Geometry check sheet. Reference: the model listing, model coordinates, mm. Face numbers are marked on the shaded views. A direction names the side the tool comes from. Round coordinates to 2 decimals unless told otherwise and drop trailing zeros. Loops run counter-clockwise (first coordinate to the right, second up) from the corner with the lowest first, then second, coordinate; pieces in that order, holes last. Notation, with made-up numbers: (-5.75, -14.5) - (5.25, -14.5) arc R16 cw to (5.25, 7.5) - close; hole circle Ø5 at (0.5, 21). An arc over 180 degrees is marked (long way). Answer as CSV lines item,"result". Start each with the question number.
1) Cross-section at A-A on x = 0. Record the boundary of the cut face in (y, z) (3 decimals), and give its area (3 significant figures).
2) Cross-section at C-C on y = -13. Record the boundary of the cut face in (x, z) (3 decimals).
3) Cross-section at B-B on z = 0. Record the boundary of the cut face in (x, y) (3 decimals), and give its area (3 significant figures).
4) Depth check by flat-ended pin: P1, Ø12, axis at x = -41.5, z = 12, coming from the +Y side; P2, Ø3, axis at y = -86, z = -41, coming from the -X side; P3, Ø4, axis at x = -43.5, z = 35.5, coming from the -Y side; P4, Ø3, axis at x = -5, y = -139, coming from the -Z side. Enter the tip coordinate at first touch or a pass-through.
5) Cross-section at D-D on x = 44. State how many separate pieces and enclosed holes the cut face has, and give its area (3 significant figures).
6) Draft check along Y on the marked faces 3, 4 and 5. Enter one of: released by +Y, released by -Y, zero draft, split by the parting line, or undercut.
7) Access from +Z, -Z, +X, -X, +Y, -Y to the whole of each face (thin tool, end or side, straight path). Record for the marked faces 1 and 2.
8) Thickness scan on line 1 along X through (y, z) = (-18, 0) (3 decimals); line 2 along X through (y, z) = (-116.2, 0) (3 decimals); line 3 along Y through (x, z) = (2, -29.5) (3 decimals). Record the ranges inside material, lowest first.
from build123d import *

# Parameters (mm, degrees)
SHELL1_T = -3.175


with BuildPart() as part:
    # Sketch1 → Revolve1 (revolve)
    with BuildSketch(Plane(origin=(0, 0, 0), x_dir=(0, 0, -1), z_dir=(1, 0, 0)), mode=Mode.PRIVATE) as revolve1_sk:
        Polygon((0, 0), (0, -164.872045256), (50.8, -164.872045256), (38.1, -117.475), (38.1, -114.3), (79.375, -25.4), (76.2, -25.4), (76.2, 0), align=None)
    revolve(revolve1_sk.sketch.rotate(Axis((0, 0, 0), (0, -1, 0)), 180), axis=Axis((0, 0, 0), (0, -1, 0)))

    # Shell1
    shell1_openings = [part.faces().sort_by_distance(p)[0] for p in [
        (0, -164.872045256, 0),
    ]]
    offset(amount=SHELL1_T, openings=shell1_openings, kind=Kind.INTERSECTION)


solid = part.part
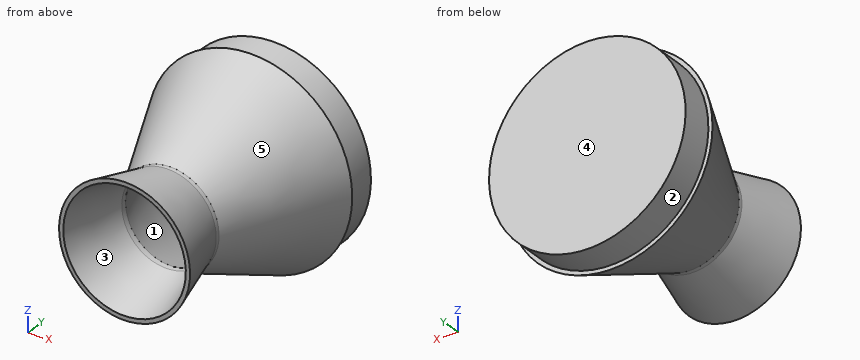
Answer block:
1,outline,"(-164.872, -50.8) - (-117.475, -38.1) - (-114.3, -38.1) - (-25.4, -79.375) - (-25.4, -76.2) - (0, -76.2) - (0, 76.2) - (-25.4, 76.2) - (-25.4, 79.375) - (-114.3, 38.1) - (-117.475, 38.1) - (-164.872, 50.8) - (-164.872, 47.513) - (-117.893, 34.925) - (-113.599, 34.925) - (-28.575, 74.4) - (-28.575, 73.025) - (-3.175, 73.025) - (-3.175, -73.025) - (-28.575, -73.025) - (-28.575, -74.4) - (-113.599, -34.925) - (-117.893, -34.925) - (-164.872, -47.513) - close"
1,area,"1,590 mm^2"
2,outline,"circle Ø152.4 at (0, 0); hole circle Ø146.05 at (0, 0)"
3,outline,"(-79.375, -25.4) - (-38.1, -114.3) - (-38.1, -117.475) - (-50.8, -164.872) - (-47.513, -164.872) - (-34.925, -117.893) - (-34.925, -113.599) - (-74.4, -28.575) - (-73.025, -28.575) - (-73.025, -3.175) - (73.025, -3.175) - (73.025, -28.575) - (74.4, -28.575) - (34.925, -113.599) - (34.925, -117.893) - (47.513, -164.872) - (50.8, -164.872) - (38.1, -117.475) - (38.1, -114.3) - (79.375, -25.4) - (76.2, -25.4) - (76.2, 0) - (-76.2, 0) - (-76.2, -25.4) - close"
3,area,"1,590 mm^2"
4,P1,"stops at y = 0"
4,P2,"stops at x = -32.94"
4,P3,"stops at y = -79.74"
4,P4,"stops at z = -44.02"
5,separate pieces,"2"
5,enclosed holes,"1"
5,area,"2,090 mm^2"
6,face 3,"released by -Y"
6,face 4,"released by +Y"
6,face 5,"undercut"
7,face 1,"none"
7,face 2,"+Y"
8,line 1,"x = -76.2 to -73.025, 73.025 to 76.2"
8,line 2,"x = -38.1 to -34.925, 34.925 to 38.1"
8,line 3,"y = -3.175 to 0"
